Could you check a few things on this model? Use its own coordinates, in mm. A direction names the side the tool comes from. Give positions to 0.01 mm unless a question says otherwise; leave off trailing zeros. Write each loop counter-clockwise with the first axis right and the second up, starting at its lowest first coordinate (ties: lowest second). Pieces come first, ordered by that corner, then holes. Notation, with made-up numbers: (48, 70) - (62, 70) arc R16 ccw to (62, 75) - close; hole circle Ø2 at (69, 56). An arc over 180 degrees is marked (long way). Answer as a JSON object with one key per item and string values. Group by question number.
```python
from build123d import *

# Parameters (mm, degrees)
FOUR_3_4_MM_POWER_PCB_SLOTS_NOMINAL_PA_DEPTH = 2.2


with BuildPart() as part:
    # Four 3.4 mm power PCB slots - nomina 2 → Four 3.4 mm power PCB slots - nominal pa (new body)
    with BuildSketch(Plane.XY):
        Polygon((-31.4, -11.4), (31.4, -11.4), (32, -10.8), (32, 10.8), (31.4, 11.4), (-31.4, 11.4), (-32, 10.8), (-32, -10.8), align=None)
        with BuildLine():
            Line((-26.1, -10.2), (-23.9, -10.2))
            ThreePointArc((-23.9, -10.2), (-22.2, -8.5), (-23.9, -6.8))
            Line((-23.9, -6.8), (-26.1, -6.8))
            ThreePointArc((-26.1, -6.8), (-27.8, -8.5), (-26.1, -10.2))
        make_face(mode=Mode.SUBTRACT)
        with BuildLine():
            Line((-26.1, 6.8), (-23.9, 6.8))
            ThreePointArc((-23.9, 6.8), (-22.2, 8.5), (-23.9, 10.2))
            Line((-23.9, 10.2), (-26.1, 10.2))
            ThreePointArc((-26.1, 10.2), (-27.8, 8.5), (-26.1, 6.8))
        make_face(mode=Mode.SUBTRACT)
        with BuildLine():
            Line((23.9, -10.2), (26.1, -10.2))
            ThreePointArc((26.1, -10.2), (27.8, -8.5), (26.1, -6.8))
            Line((26.1, -6.8), (23.9, -6.8))
            ThreePointArc((23.9, -6.8), (22.2, -8.5), (23.9, -10.2))
        make_face(mode=Mode.SUBTRACT)
        with BuildLine():
            Line((23.9, 6.8), (26.1, 6.8))
            ThreePointArc((26.1, 6.8), (27.8, 8.5), (26.1, 10.2))
            Line((26.1, 10.2), (23.9, 10.2))
            ThreePointArc((23.9, 10.2), (22.2, 8.5), (23.9, 6.8))
        make_face(mode=Mode.SUBTRACT)
    extrude(amount=FOUR_3_4_MM_POWER_PCB_SLOTS_NOMINAL_PA_DEPTH)


solid = part.part
```
(1) For faces 1 (the flat face through (25, -6.8, 1)), 2 (the flat face through (0, 11.4, 1)), which set-ups out of +Z, -Z, +X, -X, +Y, -Y let a thin tool reach every point of the face, with its end or its side?
(2) If we mould it in two halves opening along X, with no side actions, what happens to faces 3 (the flat face through (0, 0, 2.2)), 4 (the cylindrical face through (-27.8, 8.5, 1.1)), 5 (the flat face through (32, 0, 1)), 6 (the flat face through (-32, 0, 1))? For each: +X half, -X half, draft (parallel to the pull), parting line (faces both ways), or undercut.
(3) I want a section at B-B, the plane z = 0.75. Please give me the cut outline in (x, y), and give its area (3 significant figures).
(4) I need wall thicknesses on L1, parallel to X at y = 9.75, z = 1.5; L2, parallel to X at y = -7.75, z = 0.45. Which ranges of each line are inside material? Lowest first, please.
(5) I want a section at A-A, the plane y = 8. Please give me the cut outline in (x, z), and give its area (3 significant figures).
(6) I want a section at C-C, the plane y = -8.5. Please give me the cut outline in (x, z), and give its area (3 significant figures).
Entries:
{
 "1": {"face 1": "+Z, -Z", "face 2": "+Z, -Z, +X, -X, +Y"},
 "2": {"face 3": "draft", "face 4": "undercut", "face 5": "+X half", "face 6": "-X half"},
 "3": {"outline": "(-32, -10.8) - (-31.4, -11.4) - (31.4, -11.4) - (32, -10.8) - (32, 10.8) - (31.4, 11.4) - (-31.4, 11.4) - (-32, 10.8) - close; hole (-26.1, -10.2) - (-23.9, -10.2) arc R1.7 ccw to (-23.9, -6.8) - (-26.1, -6.8) arc R1.7 ccw to start; hole (-26.1, 6.8) - (-23.9, 6.8) arc R1.7 ccw to (-23.9, 10.2) - (-26.1, 10.2) arc R1.7 ccw to start; hole (23.9, -10.2) - (26.1, -10.2) arc R1.7 ccw to (26.1, -6.8) - (23.9, -6.8) arc R1.7 ccw to start; hole (23.9, 6.8) - (26.1, 6.8) arc R1.7 ccw to (26.1, 10.2) - (23.9, 10.2) arc R1.7 ccw to start", "area": "1,390 mm^2"},
 "4": {"L1": "-32 to -27.25, -22.75 to 22.75, 27.25 to 32", "L2": "-32 to -27.63, -22.37 to 22.37, 27.63 to 32"},
 "5": {"outline": "(-32, 0) - (-27.72, 0) - (-27.72, 2.2) - (-32, 2.2) - close; (-22.28, 0) - (22.28, 0) - (22.28, 2.2) - (-22.28, 2.2) - close; (27.72, 0) - (32, 0) - (32, 2.2) - (27.72, 2.2) - close", "area": "117 mm^2"},
 "6": {"outline": "(-32, 0) - (-27.8, 0) - (-27.8, 2.2) - (-32, 2.2) - close; (-22.2, 0) - (22.2, 0) - (22.2, 2.2) - (-22.2, 2.2) - close; (27.8, 0) - (32, 0) - (32, 2.2) - (27.8, 2.2) - close", "area": "116 mm^2"}
}
